```python
from build123d import *

# Parameters (mm, degrees)
EXTRUDE_1_DEPTH      = 35
EXTRUDE_1_DEPTH_BACK = 35
SKETCH_1_R           = 175
CUT_EXTRUDE_2_DEPTH  = 258.196422992
SKETCH_3_R           = 135
CUT_EXTRUDE_3_DEPTH  = 5
SKETCH_4_R           = 10
CUT_EXTRUDE_4_DEPTH  = 30


with BuildPart() as part:
    # 스케치1 → 보스-돌출1 (new, two sides: drawn at the far end of the back side and taken through both)
    with BuildSketch(Plane.XY.offset(-EXTRUDE_1_DEPTH_BACK)):
        Circle(SKETCH_1_R)
    extrude(amount=EXTRUDE_1_DEPTH + EXTRUDE_1_DEPTH_BACK)

    # 스케치2 → 컷-돌출2 (cut, through all)
    with BuildSketch(Plane.XY.offset(35)):
        with BuildLine():
            ThreePointArc((39.333286641, 102.727272727), (0, 110), (-39.333286641, 102.727272727))
            ThreePointArc((-39.333286641, 102.727272727), (0, 70), (39.333286641, 102.727272727))
        make_face()
        with BuildLine():
            ThreePointArc((-85.544788112, 69.152651626), (-104.616216792, 33.991869381), (-109.854096145, -5.663705509))
            ThreePointArc((-109.854096145, -5.663705509), (-66.573956141, 21.631189606), (-85.544788112, 69.152651626))
        make_face()
        with BuildLine():
            ThreePointArc((-92.202873255, -59.98858361), (-64.656377752, -88.991869381), (-28.56027858, -106.227635234))
            ThreePointArc((-28.56027858, -106.227635234), (-41.14496766, -56.631189606), (-92.202873255, -59.98858361))
        make_face()
        with BuildLine():
            ThreePointArc((28.56027858, -106.227635234), (64.656377752, -88.991869381), (92.202873255, -59.98858361))
            ThreePointArc((92.202873255, -59.98858361), (41.14496766, -56.631189606), (28.56027858, -106.227635234))
        make_face()
        with BuildLine():
            ThreePointArc((109.854096145, -5.663705509), (104.616216792, 33.991869381), (85.544788112, 69.152651626))
            ThreePointArc((85.544788112, 69.152651626), (66.573956141, 21.631189606), (109.854096145, -5.663705509))
        make_face()
    extrude(amount=-CUT_EXTRUDE_2_DEPTH, mode=Mode.SUBTRACT)

    # 스케치3 → 컷-돌출3 (cut)
    with BuildSketch(Plane.XY.offset(35)):
        Circle(SKETCH_3_R)
    cut_extrude_3 = extrude(amount=-CUT_EXTRUDE_3_DEPTH, mode=Mode.SUBTRACT)

    # 대칭 복사1: 컷-돌출3 across plane
    add(cut_extrude_3.mirror(Plane.XY), mode=Mode.SUBTRACT)

    # 스케치4 → 컷-돌출4 (cut)
    with BuildSketch(Plane(origin=(0, 0, -30), x_dir=(-1, 0, 0), z_dir=(0, 0, -1))):
        Circle(SKETCH_4_R)
    extrude(amount=-CUT_EXTRUDE_4_DEPTH, mode=Mode.SUBTRACT)


solid = part.part
```
Here's how the part is built. I have some questions about the finished solid (model axes, mm). A direction names the side the tool comes from. Round coordinates to 2 decimals unless told otherwise and drop trailing zeros. Loops run counter-clockwise (first coordinate to the right, second up) from the corner with the lowest first, then second, coordinate; pieces in that order, holes last.
1. Suppose I cut it at A-A, the plane x = 0. Please give me the cut outline in (y, z), and give its area (3 significant figures).
Answers:
outline: (-175, -35) - (-135, -35) - (-135, -30) - (-10, -30) - (-10, 0) - (10, 0) - (10, -30) - (70, -30) - (70, 30) - (-135, 30) - (-135, 35) - (-175, 35) - close; (110, -30) - (135, -30) - (135, -35) - (175, -35) - (175, 35) - (135, 35) - (135, 30) - (110, 30) - close
area: 18,800 mm2
2. Will these pins go through, and if not, where does the flat tip stop? pin 1 (1.5 mm diameter, centred on y = -109, z = -23, fed in from +X); pin 2 (10 mm diameter, centred on x = -37, y = -0.5, fed in from +Z); pin 3 (3 mm diameter, centred on x = -59.5, z = -1, fed in from +Y).
Answers:
pin 1: stops at x = 137.5
pin 2: stops at z = 30
pin 3: stops at y = 165.11
3. Suppose I cut it at B-B, the plane z = 22. Please give me the cut outline in (x, y).
Answers:
outline: circle Ø350 at (0, 0); hole (-109.85, -5.66) arc R40 ccw to (-85.54, 69.15) arc R110 ccw to start; hole (-92.2, -59.99) arc R110 ccw to (-28.56, -106.23) arc R40 ccw to start; hole (-39.33, 102.73) arc R40 ccw to (39.33, 102.73) arc R110 ccw to start; hole (28.56, -106.23) arc R110 ccw to (92.2, -59.99) arc R40 ccw to start; hole (85.54, 69.15) arc R40 ccw to (109.85, -5.66) arc R110 ccw to start
4. Thinking about a two-plate mould opening in X: for faces 5 (the face through (64.2, -89.32, 0.42)), 6 (the face through (90, -103, 35)), 7 (the face through (-128.982, 118.273, -0.49)), which applies, released by +X, released by -X, zero draft, split by the parting line, or undercut?
Answers:
face 5: undercut
face 6: zero draft
face 7: split by the parting line
5. If I drill on probe 1 along Y at (x, z) = (0, 32.6); probe 2 along Y at (x, z) = (0, -24); probe 3 along X at (y, z) = (30, 25.5), over which ranges is the centre line in solid material (lowest first)?
Answers:
probe 1: y = -175 to -135, 135 to 175
probe 2: y = -175 to -10, 10 to 70, 110 to 175
probe 3: x = -172.41 to -105.83, -64.82 to 64.82, 105.83 to 172.41
6. Suppose I cut it at C-C, the plane z = -24. Please give me the cut outline in (x, y).
Answers:
outline: circle Ø350 at (0, 0); hole (-109.85, -5.66) arc R40 ccw to (-85.54, 69.15) arc R110 ccw to start; hole (-92.2, -59.99) arc R110 ccw to (-28.56, -106.23) arc R40 ccw to start; hole (-39.33, 102.73) arc R40 ccw to (39.33, 102.73) arc R110 ccw to start; hole circle Ø20 at (0, 0); hole (28.56, -106.23) arc R110 ccw to (92.2, -59.99) arc R40 ccw to start; hole (85.54, 69.15) arc R40 ccw to (109.85, -5.66) arc R110 ccw to start
7. Suppose I cut it at D-D, the plane y = 78. Please give me the cut outline in (x, z).
Answers:
outline: (-156.66, -35) - (-110.19, -35) - (-110.19, -30) - (-24, -30) - (-24, 30) - (-110.19, 30) - (-110.19, 35) - (-156.66, 35) - close; (24, -30) - (110.19, -30) - (110.19, -35) - (156.66, -35) - (156.66, 35) - (110.19, 35) - (110.19, 30) - (24, 30) - close
8. For faces 1 (the face through (0.6, 110, 0.4)), 2 (the face through (90, -103, -35)), 3 (the face through (-2, 2, 30)), 4 (the face through (2.17, -9.76, -15.21)), which set-ups out of +Z, -Z, +X, -X, +Y, -Y let a thin tool reach every point of the face, with its end or its side?
Answers:
face 1: +Z, -Z
face 2: -Z, +X, -X, +Y, -Y
face 3: +Z
face 4: -Z
